Geometry check sheet. Reference: the model listing, model coordinates, mm. A direction names the side the tool comes from. Give positions to 0.01 mm unless a question says otherwise; leave off trailing zeros. Write each loop counter-clockwise with the first axis right and the second up, starting at its lowest first coordinate (ties: lowest second). Pieces come first, ordered by that corner, then holes. Notation, with made-up numbers: (50.5, 25) - (92.5, 25) arc R26 cw to (92.5, 43) - close; hole circle Ø6 at (77, 20.25). An arc over 180 degrees is marked (long way). Write item = value, one per line. Start each with the question number.
(1) Section check B-B, the plane x = 4.5. Enter the section's corners in (y, z).
(2) Thickness scan on L1, parallel to Z at x = 13, y = -3.85; L2, parallel to X at y = -0.5, z = 6; L3, parallel to X at y = -3.55, z = 17. Record the ranges inside material, lowest first.
(3) Access from +Z, -Z, +X, -X, +Y, -Y to the whole of each face (thin tool, end or side, straight path). Record for faces 1 (the cylindrical face through (-21.6, -3, 28.8)), 2 (the flat face through (17, -3, 6.35)).
(4) Section check A-A, the plane y = -3.55. Enter the section's corners in (x, z) (3 decimals).
(5) Depth check by flat-ended pin: pin 1 Ø3 at (x, y) = (16.5, -3) entering from +Z; pin 2 Ø1 at (y, z) = (-4, 16.5) entering from +X; pin 3 Ø3 at (x, y) = (-9, -4.5) entering from +Z. Enter the tip coordinate at first touch or a pass-through.
(6) Section check C-C, the plane z = 16.5. Enter the section's corners in (x, y), plus the area to 3 significant figures.
```python
from build123d import *

# Parameters (mm, degrees)
F1_DEPTH = 5.842
F2_R     = 3.175
F3_R     = 3.175


with BuildPart() as f1:
    # F0 (on Front) → F1 (new body)
    with BuildSketch(Plane.XZ):
        Polygon((31.75, 6.35), (0, 6.35), (-22.225, 31.75), (-31.75, 6.35), (-31.75, -6.35), (31.75, -6.35), align=None)
    extrude(amount=F1_DEPTH)

    # F2
    f2_edges = [f1.edges().sort_by_distance(p)[0] for p in [
        (0, -2.921, 6.35),
        (-31.75, -2.921, 6.35),
        (-31.75, -2.921, -6.35),
    ]]
    fillet(f2_edges, radius=F2_R)

    # F3
    f3_edges = [f1.edges().sort_by_distance(p)[0] for p in [
        (-22.225, -2.921, 31.75),
    ]]
    fillet(f3_edges, radius=F3_R)


solid = f1.part
```
Model answer:
q1.outline = (-5.84, -6.35) - (0, -6.35) - (0, 6.35) - (-5.84, 6.35) - close
q2.L1 = -6.35 to 6.35
q2.L2 = -31.74 to 31.75
q2.L3 = -27.76 to -9.32
q3.face_1 = +Z, +Y, -Y
q3.face_2 = +Z, +X, +Y, -Y
q4.outline = (-31.75, -3.175) arc R3.175 ccw to (-28.575, -6.35) - (31.75, -6.35) - (31.75, 6.35) - (1.441, 6.35) arc R3.175 cw to (-0.949, 7.434) - (-18.728, 27.753) arc R3.175 ccw to (-24.09, 26.777) - (-31.548, 6.889) arc R3.175 ccw to (-31.75, 5.774) - close
q5.pin_1 = 6.35
q5.pin_2 = -8.44
q5.pin_3 = 18.35
q6.outline = (-27.94, -5.84) - (-8.88, -5.84) - (-8.88, 0) - (-27.94, 0) - close
q6.area = 111 mm²
